Build history of the part. All positions in model axes, mm. A direction names the side the tool comes from. Round coordinates to 2 decimals unless told otherwise and drop trailing zeros. Loops run counter-clockwise (first coordinate to the right, second up) from the corner with the lowest first, then second, coordinate; pieces in that order, holes last. Notation, with made-up numbers: (9.25, 59.25) -> (34.25, 59.25) arc R20 ccw to (34.25, 75.25) -> close; hole circle Ø10 at (52.5, -7). An arc over 180 degrees is marked (long way). Put each result on its own line as item: value. Start each with the question number.
Item 1: Pull direction Y, two halves, no side cores. Call faces 1 (the flat face through (-18, 3, -30)), 2 (the cylindrical face through (-2.343, 17.847, -15.804)), 3 (the cylindrical face through (-2.17, 9.76, 15.8)), 4 (the flat face through (4, -12, -2)): +Y half, -Y half, draft (parallel to the pull), parting line (faces both ways), or undercut.
Item 2: Flat gauge pins, fed straight in: pin 1 Ø1 at (x, z) = (1.5, -18) entering from +Y (3 decimals); pin 2 Ø5 at (x, z) = (4, 6.5) entering from +Y; pin 3 Ø4 at (y, z) = (12, -20) entering from +X; pin 4 Ø10 at (x, y) = (13.5, -0.5) entering from +Z. Where does each tip first touch, or does it go through?
Item 3: Cut at C-C, the plane z = -12.5. List the corners of the cut face in (x, y), plus the area to 3 significant figures.
Item 4: Cut at A-A, the plane x = 0. List the corners of the cut face in (y, z), plus the area to 3 significant figures.
Item 5: Cut at D-D, the plane y = -17. List the corners of the cut face in (x, z).
Item 6: Drill centre lines: probe 1 along Y at (x, z) = (0, 10.25); probe 2 along Y at (x, z) = (0, -18); probe 3 along Z at (x, y) = (-5.5, -13.5). Where is each one in solid material? Low to high. Write a range as [from, to].
Item 7: Tool access for faces 5 (the cylindrical face through (-4.336, -19.524, -14.79)), 6 (the flat face through (9, -9, 0)): list every direction of +Z, -Z, +X, -X, +Y, -Y with a clear straight run to the whole face (end or side of a thin tool).
Autodesk Inventor part; units mm, degrees
ref_plane "YZ Plane" through (0, 0, 0) normal (1, 0, 0) x (0, 1, 0)
ref_plane "XZ Plane" through (0, 0, 0) normal (0, 1, 0) x (-1, 0, 0)
ref_plane "XY Plane" through (0, 0, 0) normal (0, 0, 1) x (1, 0, 0)
sketch "Sketch1" plane through (0, 0, 0) normal (0, 0, 1) x (1, 0, 0)
  circle A0 centre (0, 0) radius 20
  dimension "d0" = 40
extrude "Extrusion1" add sketch "Sketch1" against normal blind 30
sketch "Sketch2" plane through (0, 0, 0) normal (0, 0, 1) x (1, 0, 0)
  circle A0 centre (0, 0) radius 10
  dimension "d4" = 20
extrude "Extrusion2" add sketch "Sketch2" along normal blind 30
fillet "Fillet1" radius 2 1 edges at (-10, 0, 0)
shell "Shell1" thickness 2 removed faces 2 at (-2.364, 6.2334, -30) at (-1.182, 3.1167, 30)
Reply:
1. face 1: draft
1. face 2: undercut
1. face 3: parting line
1. face 4: undercut
2. pin 1: stops at y = 19.975
2. pin 2: stops at y = 9.89
2. pin 3: stops at x = 17.32
2. pin 4: stops at z = 30
3. outline: circle Ø40 at (0, 0); hole circle Ø36 at (0, 0)
3. area: 239 mm^2
4. outline: (-20, -30) -> (-18, -30) -> (-18, -2) -> (-12, -2) arc R4 ccw to (-8, 2) -> (-8, 30) -> (-10, 30) -> (-10, 2) arc R2 cw to (-12, 0) -> (-20, 0) -> close; (8, 2) arc R4 ccw to (12, -2) -> (18, -2) -> (18, -30) -> (20, -30) -> (20, 0) -> (12, 0) arc R2 cw to (10, 2) -> (10, 30) -> (8, 30) -> close
4. area: 275 mm^2
5. outline: (-10.54, -30) -> (-5.92, -30) -> (-5.92, -2) -> (5.92, -2) -> (5.92, -30) -> (10.54, -30) -> (10.54, 0) -> (-10.54, 0) -> close
6. probe 1: y = [-10, -8], [8, 10]
6. probe 2: y = [-20, -18], [18, 20]
6. probe 3: z = [-2, 0]
7. face 5: +Z, -Z
7. face 6: +Z
